from build123d import *

# Parameters (mm, degrees)
SKETCH1_W           = 60
SKETCH1_H           = 2.05
SKETCH1_W_2         = 47.3
SKETCH1_H_2         = 1.95
SKETCH1_W_3         = 1.27
SKETCH1_W_4         = 6.35
SKETCH2_R           = 1.5
BOSS_EXTRUDE1_DEPTH = 3
SKETCH5_R           = 1.5
CUT_EXTRUDE1_DEPTH  = 10
SKETCH6_R           = 3
SKETCH6_R_2         = 15.05
CUT_EXTRUDE2_DEPTH  = 51.92


with BuildPart() as part:
    # Sketch1 → Revolve1 (revolve)
    with BuildSketch(Plane.XY):
        with Locations((0, 18.025)):
            Rectangle(SKETCH1_W, SKETCH1_H)
        with Locations((0, 16.025)):
            Rectangle(SKETCH1_W_2, SKETCH1_H_2)
        with Locations((24.285, 16.025)):
            Rectangle(SKETCH1_W_3, SKETCH1_H_2)
        with Locations((-26.825, 16.025)):
            Rectangle(SKETCH1_W_4, SKETCH1_H_2)
    revolve(axis=Axis((0, 0, 0), (-1, 0, 0)))

    # Sketch2 → Boss-Extrude1 (add)
    with BuildSketch(Plane(origin=(24.92, 0, 0), x_dir=(0, 0, -1), z_dir=(1, 0, 0))):
        with BuildLine():
            ThreePointArc((-3.73983832, 14.577932273), (-3.194140619, 13.871382665), (-3, 13))
            ThreePointArc((-3, 13), (0, 10), (3, 13))
            ThreePointArc((3, 13), (3.194140619, 13.871382665), (3.73983832, 14.577932273))
            ThreePointArc((3.73983832, 14.577932273), (0, 15.05), (-3.73983832, 14.577932273))
        make_face()
        with Locations((0, 13)):
            Circle(SKETCH2_R, mode=Mode.SUBTRACT)
        with BuildLine():
            ThreePointArc((-9.758330249, 9.098076211), (-10.415899464, 9.701898251), (-10.754940523, 10.527761127))
            ThreePointArc((-10.754940523, 10.527761127), (-13.033682327, 7.525), (-14.494778842, 4.050171146))
            ThreePointArc((-14.494778842, 4.050171146), (-13.610040083, 4.169484414), (-12.758330249, 3.901923789))
            ThreePointArc((-12.758330249, 3.901923789), (-8.660254038, 5), (-9.758330249, 9.098076211))
        make_face()
        with Locations((-11.258330249, 6.5)):
            Circle(SKETCH2_R, mode=Mode.SUBTRACT)
        with BuildLine():
            ThreePointArc((10.754940523, -10.527761127), (13.033682327, -7.525), (14.494778842, -4.050171146))
            ThreePointArc((14.494778842, -4.050171146), (13.610040083, -4.169484414), (12.758330249, -3.901923789))
            ThreePointArc((12.758330249, -3.901923789), (8.660254038, -5), (9.758330249, -9.098076211))
            ThreePointArc((9.758330249, -9.098076211), (10.415899464, -9.701898251), (10.754940523, -10.527761127))
        make_face()
        with Locations((11.258330249, -6.5)):
            Circle(SKETCH2_R, mode=Mode.SUBTRACT)
        with BuildLine():
            ThreePointArc((-3, -13), (-3.194140619, -13.871382665), (-3.73983832, -14.577932273))
            ThreePointArc((-3.73983832, -14.577932273), (0, -15.05), (3.73983832, -14.577932273))
            ThreePointArc((3.73983832, -14.577932273), (3.194140619, -13.871382665), (3, -13))
            ThreePointArc((3, -13), (0, -10), (-3, -13))
        make_face()
        with Locations((0, -13)):
            Circle(SKETCH2_R, mode=Mode.SUBTRACT)
    extrude(amount=-BOSS_EXTRUDE1_DEPTH)

    # Sketch5 → Cut-Extrude1 (cut)
    with BuildSketch(Plane.ZY.offset(30)):
        with Locations((-8.525, -14.765733135)):
            Circle(SKETCH5_R)
        with Locations((8.525, -14.765733135)):
            Circle(SKETCH5_R)
        with Locations((17.05, 0)):
            Circle(SKETCH5_R)
        with Locations((-17.05, 0)):
            Circle(SKETCH5_R)
        with Locations((8.525, 14.765733135)):
            Circle(SKETCH5_R)
        with Locations((-8.525, 14.765733135)):
            Circle(SKETCH5_R)
    extrude(amount=-CUT_EXTRUDE1_DEPTH, mode=Mode.SUBTRACT)

    # Sketch6 → Cut-Extrude2 (cut)
    with BuildSketch(Plane.ZY.offset(30)):
        with Locations((-11.258330249, 6.5)):
            Circle(SKETCH6_R)
        Circle(SKETCH6_R_2)
        with Locations((-11.258330249, 6.5)):
            Circle(SKETCH6_R)
        Circle(SKETCH6_R_2)
        with Locations((0, 13)):
            Circle(SKETCH6_R)
        Circle(SKETCH6_R_2)
        with Locations((11.258330249, 6.5)):
            Circle(SKETCH6_R)
        Circle(SKETCH6_R_2)
        with Locations((11.258330249, 6.5)):
            Circle(SKETCH6_R)
        Circle(SKETCH6_R_2)
        with Locations((11.258330249, -6.5)):
            Circle(SKETCH6_R)
        Circle(SKETCH6_R_2)
        with Locations((11.258330249, -6.5)):
            Circle(SKETCH6_R)
        Circle(SKETCH6_R_2)
        with Locations((0, -13)):
            Circle(SKETCH6_R)
        Circle(SKETCH6_R_2)
        with Locations((0, -13)):
            Circle(SKETCH6_R)
        Circle(SKETCH6_R_2)
        with Locations((-11.258330249, -6.5)):
            Circle(SKETCH6_R)
        Circle(SKETCH6_R_2)
        with Locations((-11.258330249, -6.5)):
            Circle(SKETCH6_R)
        Circle(SKETCH6_R_2)
    extrude(amount=-CUT_EXTRUDE2_DEPTH, mode=Mode.SUBTRACT)


solid = part.part
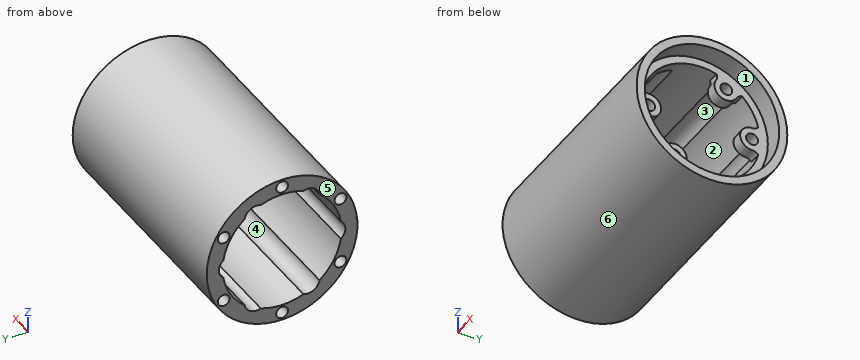
The model under review builds one solid part; all positions refer to its coordinate system, in mm. Face numbers are marked on the shaded views. A direction names the side the tool comes from. Give positions to 0.01 mm unless a question says otherwise; leave off trailing zeros. Order: outer loops, then holes, each group sorted by start corner. A loop starts at its lowest first (then second) coordinate and runs counter-clockwise, first axis right, second up. Notation, with made-up numbers: M 60.25,-38.75 L 84.25,-38.75 A19 cw 84.25,-20.75 Z; hole C 4.5,-17.75 d7. An arc over 180 degrees is marked long. Use one line per item in the form item = value. Start each with the question number.
Item 1: We need section D-D on x = 6. Give the boundary of the cut face in (y, z).
Item 2: We need section C-C on z = -6. Give the boundary of the cut face in (x, y).
Item 3: For the marked faces 1 and 2, list the 3-axis set-ups (+Z, -Z, +X, -X, +Y, -Y) from which the entire face can be reached by the end or side of a thin tool; tool diameter is ignored.
Item 4: Insertion check: pin 1 Ø5 at (y, z) = (-6.5, -11.26) entering from +X; pin 2 Ø3 at (y, z) = (-6, -12) entering from -X; pin 3 Ø3 at (x, y) = (-10, 10) entering from -Z. Each pin has a flat end and moves straight along its axis. Give the tip position at first contact, or say it passes through.
Item 5: To check wall thickness, follow line 1 along Z through (x, y) = (10.5, 6.5); line 2 along Y through (x, z) = (27.8, 0); line 3 along Z through (x, y) = (-10.5, 11). State the ranges of each line that lie inside material, in increasing order. Write a range as from..to.
Item 6: We need section B-B on y = 0. Give the boundary of the cut face in (x, z), plus the area to 3 significant figures.
Item 7: We need section A-A on z = 0. Give the boundary of the cut face in (x, y), plus the area to 3 significant figures.
Item 8: The part is to be moulded in two halves that separate along Y. For the marked faces 3, 4, 5 and 6, say which applies: pulls with the +Y half, pulls with the -Y half, needs draft (parallel to the pull), parting line crosses it, or undercut.
Completed:
q1.outline = C 0,0 d38.1; hole M -14.87,-2.35 A15.05 ccw -9.47,-11.7 A3 ccw -5.4,-14.05 A15.05 ccw 5.4,-14.05 A3 ccw 9.47,-11.7 A15.05 ccw 14.87,-2.35 A3 ccw 14.87,2.35 A15.05 ccw 9.47,11.7 A3 ccw 5.4,14.05 A15.05 ccw -5.4,14.05 A3 ccw -9.47,11.7 A15.05 ccw -14.87,2.35 A3 ccw Z
q2.outline = M -30,-18.08 L 30,-18.08 L 30,-15.91 L 24.92,-15.91 L 24.92,-13.8 L -30,-13.8 Z; M -30,13.8 L 24.92,13.8 L 24.92,15.91 L 30,15.91 L 30,18.08 L -30,18.08 Z
q3.face_1 = +X
q3.face_2 = -X
q4.pin_1 = 24.92
q4.pin_2 = 21.92
q4.pin_3 = -17.05
q5.line_1 = -17.91..-14.26, 14.26..17.91
q5.line_2 = -19.05..-17, 17..19.05
q5.line_3 = -15.55..-10.27, 10.27..15.55
q6.outline = M -30,-19.05 L 30,-19.05 L 30,-17 L 24.92,-17 L 24.92,-15.05 L -30,-15.05 L -30,-15.55 L -20,-15.55 L -20,-18.55 L -30,-18.55 Z; M -30,15.05 L 24.92,15.05 L 24.92,17 L 30,17 L 30,19.05 L -30,19.05 L -30,18.55 L -20,18.55 L -20,15.55 L -30,15.55 Z
q6.area = 400 mm²
q7.outline = M -30,-19.05 L 30,-19.05 L 30,-17 L 24.92,-17 L 24.92,-14.5 L 21.92,-14.5 L 21.92,-16 L -30,-16 Z; M -30,16 L 21.92,16 L 21.92,14.5 L 24.92,14.5 L 24.92,17 L 30,17 L 30,19.05 L -30,19.05 Z; M 21.92,-11.5 L 24.92,-11.5 L 24.92,-10 L 21.92,-10 Z; M 21.92,10 L 24.92,10 L 24.92,11.5 L 21.92,11.5 Z
q7.area = 374 mm²
q8.face_3 = undercut
q8.face_4 = undercut
q8.face_5 = needs draft
q8.face_6 = parting line crosses it
